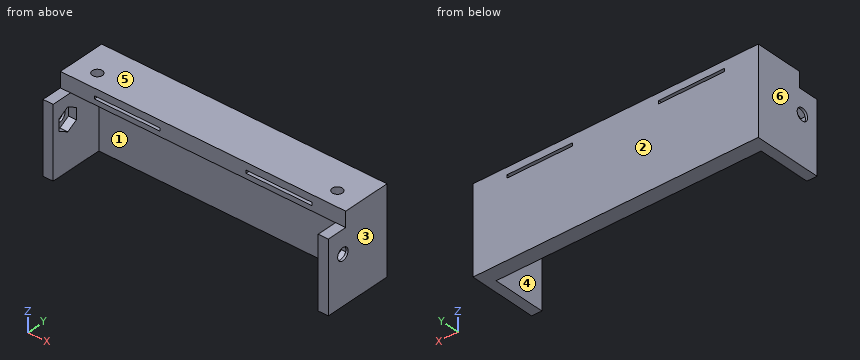
```python
from build123d import *

# Parameters (mm, degrees)
SCHIZZO1_W                   = 56.4
SCHIZZO1_H                   = 9.5
SCHIZZO1_R                   = 1
ESTRUSIONE_ESTRUSIONE1_DEPTH = 3
SCHIZZO2_W                   = 56.4
SCHIZZO2_H                   = 3
ESTRUSIONE_ESTRUSIONE2_DEPTH = 14
SCHIZZO3_W                   = 14
SCHIZZO3_H                   = 10.5
ESTRUSIONE_ESTRUSIONE3_DEPTH = 2
FORO_PER_VITE_M2_1_D         = 2.4
FORO_PER_VITE_M2_1_DEPTH     = 56.4
TAGLIO_ESTRUSIONE1_DEPTH     = 1.56
TAGLIO_ESTRUSIONE3_START     = -9.5
SCHIZZO8_W                   = 13
SCHIZZO8_H                   = 0.6
TAGLIO_ESTRUSIONE3_DEPTH     = 9.5


with BuildPart() as part:
    # Schizzo1 → Estrusione-Estrusione1 (new body)
    with BuildSketch(Plane.XY):
        with Locations((0, -4.75)):
            Rectangle(SCHIZZO1_W, SCHIZZO1_H)
        with Locations((-23.725, -6.2)):
            Circle(SCHIZZO1_R, mode=Mode.SUBTRACT)
        with Locations(Location((23.725, -6.2, 0), (0, 0, 180))):
            Circle(SCHIZZO1_R, mode=Mode.SUBTRACT)
    extrude(amount=ESTRUSIONE_ESTRUSIONE1_DEPTH)

    # Schizzo2 → Estrusione-Estrusione2 (add)
    with BuildSketch(Plane(origin=(0, 0, 0), x_dir=(-1, 0, 0), z_dir=(0, 0, -1))):
        with Locations((0, -1.5)):
            Rectangle(SCHIZZO2_W, SCHIZZO2_H)
    extrude(amount=ESTRUSIONE_ESTRUSIONE2_DEPTH)

    # Schizzo3 → Estrusione-Estrusione3 (add)
    with BuildSketch(Plane(origin=(28.2, 0, 0), x_dir=(0, 0, -1), z_dir=(1, 0, 0))):
        with Locations((7, -8.25)):
            Rectangle(SCHIZZO3_W, SCHIZZO3_H)
    estrusione_estrusione3 = extrude(amount=-ESTRUSIONE_ESTRUSIONE3_DEPTH)

    # Foro per Vite M2-1
    with Locations(Plane(origin=(28.2, 0, 0), x_dir=(0, 0, -1), z_dir=(1, 0, 0))):
        with Locations((4.5, -10.14)):
            foro_per_vite_m2_1 = Hole(FORO_PER_VITE_M2_1_D / 2, depth=FORO_PER_VITE_M2_1_DEPTH)

    # Schizzo6 → Taglio-Estrusione1 (cut)
    with BuildSketch(Plane.ZY.offset(-26.2)):
        Polygon((-5.640266782, -8.165), (-6.780533563, -10.14), (-5.640266782, -12.115), (-3.359733218, -12.115), (-2.219466437, -10.14), (-3.359733218, -8.165), align=None)
    taglio_estrusione1 = extrude(amount=-TAGLIO_ESTRUSIONE1_DEPTH, mode=Mode.SUBTRACT)

    # Specchia2: Estrusione-Estrusione3, Foro per Vite M2-1, Taglio-Estrusione1 across plane
    add(estrusione_estrusione3.mirror(Plane(origin=(0, 0, 0), x_dir=(0, 0, 1), z_dir=(1, 0, 0))))
    add(foro_per_vite_m2_1.mirror(Plane(origin=(0, 0, 0), x_dir=(0, 0, 1), z_dir=(1, 0, 0))), mode=Mode.SUBTRACT)
    add(taglio_estrusione1.mirror(Plane(origin=(0, 0, 0), x_dir=(0, 0, 1), z_dir=(1, 0, 0))), mode=Mode.SUBTRACT)

    # Schizzo8 → Taglio-Estrusione3 (cut)
    with BuildSketch(Plane(origin=(0, 0, -9), x_dir=(1, 0, 0), z_dir=(0, 1, 0)).offset(TAGLIO_ESTRUSIONE3_START)):
        with Locations((15, -10.3)):
            Rectangle(SCHIZZO8_W, SCHIZZO8_H)
        with Locations((-15, -10.3)):
            Rectangle(SCHIZZO8_W, SCHIZZO8_H)
    extrude(amount=TAGLIO_ESTRUSIONE3_DEPTH, mode=Mode.SUBTRACT)


solid = part.part
```
Input: part model. Units: mm. Frame: model coordinates. Face numbers are marked on the shaded views. A direction names the side the tool comes from. Give positions to 0.01 mm unless a question says otherwise; leave off trailing zeros. Write each loop counter-clockwise with the first axis right and the second up, starting at its lowest first coordinate (ties: lowest second). Pieces come first, ordered by that corner, then holes. Notation, with made-up numbers: (6.25, 5.25) - (24.25, 5.25) arc R23 cw to (24.25, 30.25) - close; hole circle Ø10 at (-14, 86). An arc over 180 degrees is marked (long way). Write item = value, one per line. Start each with the question number.
1. Mould query, pull axis X, two halves, no side actions, for the marked faces 3, 4, 5 and 6. Classes: released by +X, released by -X, zero draft, split by the parting line, or undercut.
2. Section query B-B, the plane z = -4.5. Output: boundary loops of the cut face in (x, y) (3 decimals), then the cut area to 3 significant figures.
3. Access query for the marked faces 1 and 2. Directions: +Z, -Z, +X, -X, +Y, -Y. A direction counts if a zero-diameter tool reaches every point of the face in a straight line with its end or side. Return the directions, or none.
4. Section query D-D, the plane x = 12.5. Output: boundary loops of the cut face in (y, z), then the cut area to 3 significant figures.
5. Section query A-A, the plane y = -6.2. Output: boundary loops of the cut face in (x, z) (3 decimals).
6. First-contact query: pin 1 Ø0.6 at (x, y) = (27.5, -11) entering from +Z; pin 2 Ø1 at (x, y) = (9, -11.5) entering from +Z; pin 3 Ø3 at (x, y) = (-1.5, -5.5) entering from -Z; pin 4 Ø3 at (x, z) = (-9.5, -4) entering from +Y. Flat tips, straight axial feed; report the tip coordinate or a pass-through.
7. Ray query, L1, parallel to X at y = -12.5, z = -3.25; L2, parallel to Y at x = -27.95, z = -4.5; L3, parallel to Z at x = 20.5, y = -5. Return the intervals inside material, ascending.
8. Section query C-C, the plane y = -2.5. Output: boundary loops of the cut face in (x, z), then the cut area to 3 significant figures.
Check sheet entries:
q1.face_3 = released by +X
q1.face_4 = undercut
q1.face_5 = zero draft
q1.face_6 = released by -X
q2.outline = (-28.2, -13.5) - (-26.2, -13.5) - (-26.2, -12.115) - (-27.76, -12.115) - (-27.76, -11.34) - (-28.2, -11.34) - close; (-28.2, -8.94) - (-27.76, -8.94) - (-27.76, -8.165) - (-26.2, -8.165) - (-26.2, -3) - (26.2, -3) - (26.2, -8.165) - (27.76, -8.165) - (27.76, -8.94) - (28.2, -8.94) - (28.2, 0) - (-28.2, 0) - close; (26.2, -13.5) - (28.2, -13.5) - (28.2, -11.34) - (27.76, -11.34) - (27.76, -12.115) - (26.2, -12.115) - close
q2.area = 197 mm2
q3.face_1 = -Z, -Y
q3.face_2 = +Z, -Z, +X, -X, +Y
q4.outline = (-9.5, 0) - (-3, 0) - (-3, -14) - (0, -14) - (0, 1) - (-9.5, 1) - close; (-9.5, 1.6) - (0, 1.6) - (0, 3) - (-9.5, 3) - close
q4.area = 64.8 mm2
q5.outline = (-28.2, -14) - (-26.2, -14) - (-26.2, 0) - (-24.725, 0) - (-24.725, 3) - (-28.2, 3) - close; (-22.725, 0) - (22.725, 0) - (22.725, 3) - (-22.725, 3) - close; (24.725, 0) - (26.2, 0) - (26.2, -14) - (28.2, -14) - (28.2, 3) - (24.725, 3) - close; hole (-21.5, 1) - (-8.5, 1) - (-8.5, 1.6) - (-21.5, 1.6) - close; hole (8.5, 1) - (21.5, 1) - (21.5, 1.6) - (8.5, 1.6) - close
q6.pin_1 = 0
q6.pin_2 = through
q6.pin_3 = 0
q6.pin_4 = 0
q7.L1 = -28.2 to -26.2, 26.2 to 28.2
q7.L2 = -13.5 to -11.34, -8.94 to 0
q7.L3 = 0 to 1, 1.6 to 3
q8.outline = (-28.2, -14) - (28.2, -14) - (28.2, 3) - (-28.2, 3) - close; hole (-21.5, 1) - (-8.5, 1) - (-8.5, 1.6) - (-21.5, 1.6) - close; hole (8.5, 1) - (21.5, 1) - (21.5, 1.6) - (8.5, 1.6) - close
q8.area = 943 mm2
